The listing builds one solid part. Answer for the finished solid, in the listing's coordinates (mm). A direction names the side the tool comes from. Round coordinates to 2 decimals unless told otherwise and drop trailing zeros. Write each loop counter-clockwise with the first axis right and the second up, starting at its lowest first coordinate (ties: lowest second). Pieces come first, ordered by that corner, then holes.
from build123d import *

# Parameters (mm, degrees)
EXTRUDE_1_DEPTH     = 15
SKETCH_5_R          = 10.1
CUT_EXTRUDE_2_DEPTH = 2


with BuildPart() as part:
    # ｽｹｯﾁ4 → ﾎﾞｽ - 押し出し1 (new body)
    with BuildSketch(Plane.XY):
        with BuildLine():
            Line((-53.623111018, -124.995132678), (-58.940636287, -129.45706617))
            ThreePointArc((-58.940636287, -129.45706617), (-60.005384698, -131.552012131), (-59.233530865, -133.771635843))
            ThreePointArc((-59.233530865, -133.771635843), (57.362306223, -135.763481103), (52.076178918, -19.270504783))
            Line((52.076178918, -19.270504783), (10.606601718, 10.606601718))
            ThreePointArc((10.606601718, 10.606601718), (-10.606601718, 10.606601718), (-10.606601718, -10.606601718))
            Line((-10.606601718, -10.606601718), (14.536280154, -62.889638219))
            ThreePointArc((14.536280154, -62.889638219), (14.918089499, -66.109676181), (13.244185189, -68.886809092))
            Line((13.244185189, -68.886809092), (-53.623111018, -124.995132678))
        make_face()
        with BuildLine():
            Line((21.232400696, -76.813798404), (45.844843506, -127.993820346))
            ThreePointArc((45.844843506, -127.993820346), (46.221944165, -131.235480845), (44.518718993, -134.019289696))
            ThreePointArc((44.518718993, -134.019289696), (-2.231208213, -149.964431749), (-47.870174388, -131.072951785))
            ThreePointArc((-47.870174388, -131.072951785), (-48.817477846, -128.802229421), (-47.747678417, -126.586582094))
            Line((-47.747678417, -126.586582094), (13.511229465, -75.151532228))
            ThreePointArc((13.511229465, -75.151532228), (17.77869109, -74.092739753), (21.232400696, -76.813798404))
        make_face(mode=Mode.SUBTRACT)
    extrude(amount=EXTRUDE_1_DEPTH)

    # ｽｹｯﾁ5 → ｶｯﾄ - 押し出し2 (cut)
    with BuildSketch(Plane.XY.offset(15)):
        Circle(SKETCH_5_R)
    extrude(amount=-CUT_EXTRUDE_2_DEPTH, mode=Mode.SUBTRACT)


solid = part.part
1. Section C-C on y = -85 is taken. Determine the outline of the cut face in (x, z).
Geometry says:
outline: (-5.96, 0) - (1.78, 0) - (1.78, 15) - (-5.96, 15) - close; (25.17, 0) - (79.84, 0) - (79.84, 15) - (25.17, 15) - close
2. For a pull along X with two mould halves and no side action, classify faces 6 (the face through (9.634, 3.034, 14.014)), 7 (the face through (25, -71, 0)), 8 (the face through (56.07, -137.06, 7.4)) as released by +X, released by -X, zero draft, split by the parting line, or undercut.
Geometry says:
face 6: undercut
face 7: zero draft
face 8: split by the parting line
3. Section D-D on x = 3 is taken. Determine the outline of the cut face in (y, z).
Geometry says:
outline: (-159.94, 0) - (-149.94, 0) - (-149.94, 15) - (-159.94, 15) - close; (-83.98, 0) - (-77.48, 0) - (-77.48, 15) - (-83.98, 15) - close; (-38.9, 0) - (14.7, 0) - (14.7, 15) - (9.64, 15) - (9.64, 13) - (-9.64, 13) - (-9.64, 15) - (-38.9, 15) - close
4. Straight lines are drawn through the part: line 1 along Y through (x, z) = (-5.5, 12.75); line 2 along Y through (x, z) = (-13.5, 12.25); line 3 along Y through (x, z) = (0, 14.15). For each, find the intervals that lie inside material, in ascending order.
Geometry says:
line 1: y = -159.81 to -149.78, -91.11 to -84.62, -21.23 to 13.96
line 2: y = -158.85 to -148.69, -97.83 to -91.33, -6.54 to 6.54
line 3: y = -160 to -150, -86.5 to -80, -32.66 to -10.1, 10.1 to 15
5. A tool of negligible diameter and unlimited length cuts with its end or side. For faces 1 (the face through (1.79, -36.38, 7.4)), 2 (the face through (-48.82, -128.84, 7.4)), 3 (the face through (0, 0, 13)), 4 (the face through (31.63, -4.54, 7.4)), 5 (the face through (25, -71, 15)), from which of +Z, -Z, +X, -X, +Y, -Y can it reach the whole face along a straight path? Write none if from no direction.
Geometry says:
face 1: +Z, -Z, -X
face 2: +Z, -Z
face 3: +Z
face 4: +Z, -Z, +X, +Y
face 5: +Z, +X, -X, +Y, -Y
6. Section B-B on x = -41 is taken. Determine the outline of the cut face in (y, z), plus the area to 3 significant figures.
Geometry says:
outline: (-148.69, 0) - (-136.74, 0) - (-136.74, 15) - (-148.69, 15) - close; (-120.92, 0) - (-114.4, 0) - (-114.4, 15) - (-120.92, 15) - close
area: 277 mm2
7. Section A-A on z = 4.5 is taken. Determine the outline of the cut face in (x, y).
Geometry says:
outline: (-59.23, -133.77) arc R80 ccw (long way) to (52.08, -19.27) - (10.61, 10.61) arc R15 ccw to (-10.61, -10.61) - (14.54, -62.89) arc R5 cw to (13.24, -68.89) - (-58.94, -129.46) arc R3 ccw to start; hole (-47.87, -131.07) arc R70 ccw to (44.52, -134.02) arc R5 ccw to (45.84, -127.99) - (21.23, -76.81) arc R5 ccw to (13.51, -75.15) - (-47.75, -126.59) arc R3 ccw to start
8. Given pin 1 (1.5 mm diameter, centred on x = -14, z = 8, fed in from +Y); pin 2 (6 mm diameter, centred on x = 4.5, y = 4, fed in from +Z); pin 3 (3 mm diameter, centred on x = -8, z = 13, fed in from +Y), each flat-ended and moving along its own axis, determine where each tip first touches the part or whether it passes through.
Geometry says:
pin 1: stops at y = 7.03
pin 2: stops at z = 13
pin 3: stops at y = 13.52
